```python
from build123d import *

# Parameters (mm, degrees)
SKETCH1_R               = 3.25
EXTRUDE1_DEPTH          = 10
SKETCH2_R               = 3.6
EXTRUDE2_DEPTH          = 6.5
SKETCH3_R               = 3.25
EXTRUDE3_DEPTH          = 3
SKETCH4_R               = 3.625
EXTRUDE4_DEPTH          = 2
SKETCH5_R               = 4.125
EXTRUDE5_DEPTH          = 6.35
SKETCH6_R               = 4
EXTRUDE6_DEPTH          = 5.75
EXTRUDE6_TAPER          = 15
SKETCH7_R               = 1.125
EXTRUDE7_DEPTH          = 0.5
EXTRUDE7_TAPER          = 15
SKETCH8_W               = 0.254
SKETCH8_H               = 4.684061481
CUT_EXTRUDE_THIN2_DEPTH = 0.5
SKETCH9_W               = 3.205351329
SKETCH9_H               = 0.254
CUT_EXTRUDE_THIN3_DEPTH = 0.5
CHAMFER1_SIZE           = 0.4
SKETCH10_R              = 0.9
CUT_EXTRUDE1_DEPTH      = 34.1
CUT_EXTRUDE1_DRAFT      = -0.5


with BuildPart() as part:
    # Sketch1 → Extrude1 (new body)
    with BuildSketch(Plane.XY):
        Circle(SKETCH1_R)
    extrude(amount=EXTRUDE1_DEPTH)

    # Sketch2 → Extrude2 (add)
    with BuildSketch(Plane.XY.offset(10)):
        with Locations(Location((0, 0, 0), (0, 0, 180))):
            Circle(SKETCH2_R)
    extrude(amount=EXTRUDE2_DEPTH)

    # Sketch3 → Extrude3 (add)
    with BuildSketch(Plane.XY.offset(16.5)):
        Circle(SKETCH3_R)
    extrude(amount=EXTRUDE3_DEPTH)

    # Sketch4 → Extrude4 (add)
    with BuildSketch(Plane.XY.offset(19.5)):
        Circle(SKETCH4_R)
    extrude(amount=EXTRUDE4_DEPTH)

    # Sketch5 → Extrude5 (add)
    with BuildSketch(Plane.XY.offset(21.5)):
        Circle(SKETCH5_R)
    extrude(amount=EXTRUDE5_DEPTH)

    # Sketch6 → Extrude6 (add)
    with BuildSketch(Plane.XY.offset(27.85)):
        Circle(SKETCH6_R)
    extrude(amount=EXTRUDE6_DEPTH, taper=EXTRUDE6_TAPER)

    # Sketch7 → Extrude7 (add)
    with BuildSketch(Plane.XY.offset(33.6)):
        Circle(SKETCH7_R)
    extrude(amount=EXTRUDE7_DEPTH, taper=EXTRUDE7_TAPER)

    # Sketch8 → Cut-Extrude-Thin2 (cut)
    with BuildSketch(Plane.XY.offset(34.1)):
        with Locations((0, -0.157007647)):
            Rectangle(SKETCH8_W, SKETCH8_H)
    extrude(amount=-CUT_EXTRUDE_THIN2_DEPTH, mode=Mode.SUBTRACT)

    # Sketch9 → Cut-Extrude-Thin3 (cut)
    with BuildSketch(Plane.XY.offset(34.1)):
        with Locations((-0.477675664, 0)):
            Rectangle(SKETCH9_W, SKETCH9_H)
    extrude(amount=-CUT_EXTRUDE_THIN3_DEPTH, mode=Mode.SUBTRACT)

    # Chamfer1
    # the kernel refuses this chamfer: 0.4 mm, written as the material it adds along each edge
    with BuildSketch(Plane(origin=(0, 0, 16.5), x_dir=(1, 0, 0), z_dir=(0, -1, 0))) as chamfer1_piece_1_section:
        Polygon((3.25, CHAMFER1_SIZE), (3.25 + CHAMFER1_SIZE, 0), (3.25, 0), align=None)
    chamfer1_piece_1 = revolve(axis=Axis((0, 0, 16.5), (0, 0, 1)), mode=Mode.PRIVATE)
    chamfer1_piece_1 = chamfer1_piece_1 & Plane(origin=(0, 0, 16.722023518), x_dir=(-1, 0, 0), z_dir=(0, 0, -1)) * Cylinder(3.6, 15, mode=Mode.PRIVATE)
    add(chamfer1_piece_1)
    with BuildSketch(Plane(origin=(0, 0, 10), x_dir=(1, 0, 0), z_dir=(0, -1, 0))) as chamfer1_piece_2_section:
        Polygon((3.25 + CHAMFER1_SIZE, 0), (3.25, -CHAMFER1_SIZE), (3.25, 0), align=None)
    chamfer1_piece_2 = revolve(axis=Axis((0, 0, 10), (0, 0, 1)), mode=Mode.PRIVATE)
    chamfer1_piece_2 = chamfer1_piece_2 & Plane(origin=(0, 0, 9.777976482), x_dir=(-1, 0, 0), z_dir=(0, 0, -1)) * Cylinder(3.6, 15, mode=Mode.PRIVATE)
    add(chamfer1_piece_2)
    # the kernel refuses this chamfer: 0.4 mm, written as the material it takes off along each edge
    with BuildSketch(Plane(origin=(0, 0, 0), x_dir=(1, 0, 0), z_dir=(0, -1, 0))) as chamfer1_2_piece_1:
        Polygon((3.25, CHAMFER1_SIZE), (3.25 - CHAMFER1_SIZE, 0), (3.25, 0), align=None)
    revolve(axis=Axis((0, 0, 0), (0, 0, 1)), mode=Mode.SUBTRACT)


with BuildPart() as cut_extrude1_tool:
    # Sketch10 → Cut-Extrude1 (with draft: the straight prism first)
    with BuildSketch(Plane(origin=(0, 0, 0), x_dir=(-1, 0, 0), z_dir=(0, 0, -1))):
        Circle(SKETCH10_R)
    extrude(amount=-CUT_EXTRUDE1_DEPTH)
    # Cut-Extrude1: the draft: its side faces are tilted about the plane it starts from
    cut_extrude1_sides = [cut_extrude1_tool.faces().sort_by_distance(p)[0] for p in [
        (0.9, 0, 17.05),
    ]]
    draft(cut_extrude1_sides, Plane(origin=(0, 0, 0), x_dir=(-1, 0, 0), z_dir=(0, 0, -1)), CUT_EXTRUDE1_DRAFT)


with BuildPart() as part_1:
    add(part.part)

    # Cut-Extrude1: cut by cut_extrude1_tool
    add(cut_extrude1_tool.part, mode=Mode.SUBTRACT)


solid = part_1.part
```
Source: CAD feature listing. Evaluate the final solid. Frame: model axes, mm. A direction names the side the tool comes from. Round coordinates to 2 decimals unless told otherwise and drop trailing zeros. Order: outer loops, then holes, each group sorted by start corner. A loop starts at its lowest first (then second) coordinate and runs counter-clockwise, first axis right, second up. Notation, with made-up numbers: (55, 29.25) -> (61, 29.25) arc R29 ccw to (61, 50.25) -> close; hole circle Ø8 at (16.5, 24.25). An arc over 180 degrees is marked (long way). One line per item, written item: value. Start each with the question number.
Q1. Section query A-A (z = 23). Return the cut outline in (x, y) (3 decimals).
Q2. Access query for faces 1 (the flat face through (-0.56, 0.56, 34.1)), 2 (the conical face through (-0.719, 0.226, 16.811)). Directions: +Z, -Z, +X, -X, +Y, -Y. A direction counts if a zero-diameter tool reaches every point of the face in a straight line with its end or side. Return the directions, or none.
Q3. Section query B-B (z = 27). Return the cut outline in (x, y) (3 decimals).
Q4. Material intervals for probe 1 along X at (y, z) = (0.5, 20); probe 2 along Y at (x, z) = (0.5, 25); probe 3 along Z at (x, y) = (-1.25, 0.5), sorted ascending.
Q5. Pin query (flat end, axial travel): pin 1 (0.6 mm diameter, centred on y = -1, z = 34, fed in from +X); pin 2 (3 mm diameter, centred on y = -0.5, z = 19, fed in from +X) (3 decimals); pin 3 (0.6 mm diameter, centred on y = -1, z = 34, fed in from -X). Return the tip coordinate at first contact, or that it passes through.
Findings below:
1. outline: circle Ø8.25 at (0, 0); hole circle Ø1.399 at (0, 0)
2. face 1: +Z, +X, -X, +Y, -Y
2. face 2: -Z
3. outline: circle Ø8.25 at (0, 0); hole circle Ø1.329 at (0, 0)
4. probe 1: -3.59 to -0.53, 0.53 to 3.59
4. probe 2: -4.09 to -0.46, 0.46 to 4.09
4. probe 3: 0 to 33.6
5. pin 1: x = 0.76
5. pin 2: x = 3.625
5. pin 3: x = -0.76
